The listing builds one solid part. Answer for the finished solid, in the listing's coordinates (mm). Give positions to 0.01 mm unless a question says otherwise; leave off trailing zeros. Order: outer loops, then holes, each group sorted by start corner. A loop starts at its lowest first (then second) coordinate and runs counter-clockwise, first axis right, second up. Notation, with made-up numbers: M 29.25,24.25 L 65.25,24.25 A15 ccw 65.25,46.25 Z; hole C 65.5,81.5 d1. An arc over 180 degrees is marked long. Answer as a JSON object with one key per item and string values. Group by question number.
```python
from build123d import *

# Parameters (mm, degrees)
SKETCH_1_R      = 0.4
EXTRUDE_1_DEPTH = 10
SKETCH_2_W      = 80
SKETCH_2_H      = 0.8
EXTRUDE_2_DEPTH = 0.8
FILLET_1_R      = 0.4
SKETCH_3_R      = 0.4
EXTRUDE_3_DEPTH = 4
SKETCH_4_R      = 0.4
EXTRUDE_4_DEPTH = 4


with BuildPart() as part:
    # 草图1 → 凸台-拉伸1 (new body)
    with BuildSketch(Plane(origin=(0, 0, 0), x_dir=(1, 0, 0), z_dir=(0, 1, 0))):
        with Locations(Location((0, 0, 0), (0, 0, 270))):
            Circle(SKETCH_1_R)
    extrude(amount=EXTRUDE_1_DEPTH)

    # 草图2 → 凸台-拉伸2 (add)
    with BuildSketch(Plane(origin=(0, 10, 0), x_dir=(1, 0, 0), z_dir=(0, 1, 0))):
        Rectangle(SKETCH_2_W, SKETCH_2_H)
    extrude(amount=EXTRUDE_2_DEPTH)

    # 圆角1
    fillet_1_edges = [part.edges().sort_by_distance(p)[0] for p in [
        (40, 10, 0),
        (40, 10.8, 0),
        (-40, 10, 0),
        (-40, 10.8, 0),
    ]]
    fillet(fillet_1_edges, radius=FILLET_1_R - 0.0001)  # a hair under: the kernel refuses the full size

    # 草图3 → 凸台-拉伸3 (add)
    with BuildSketch(Plane.XY.offset(0.4)):
        with Locations((39.6, 10.4)):
            Circle(SKETCH_3_R)
    extrude(amount=EXTRUDE_3_DEPTH)

    # 草图4 → 凸台-拉伸4 (add)
    with BuildSketch(Plane(origin=(0, 0, -0.4), x_dir=(-1, 0, 0), z_dir=(0, 0, -1))):
        with Locations((39.6, 10.4)):
            Circle(SKETCH_4_R)
    extrude(amount=EXTRUDE_4_DEPTH)

    # 草图5 → 旋转1 (revolve)
    with BuildSketch(Plane(origin=(0, 10.4, 0), x_dir=(1, 0, 0), z_dir=(0, 1, 0))):
        Polygon((39.6, -4.4), (39.6, -5.4), (40, -4.4), align=None)
    revolve(axis=Axis((39.6, 10.4, 4.4), (0, 0, 1)))

    # 草图6 → 旋转2 (revolve)
    with BuildSketch(Plane(origin=(0, 10.4, 0), x_dir=(1, 0, 0), z_dir=(0, 1, 0))):
        Polygon((-39.6, 4.4), (-39.6, 5.4), (-40, 4.4), align=None)
    revolve(axis=Axis((-39.6, 10.4, -4.4), (0, 0, -1)))


solid = part.part
```
Item 1: Section C-C (y = 2.5) is taken. Determine the outline of the cut face in (x, z), and give its area (3 significant figures).
Item 2: Consider probe 1 along Y at (x, z) = (4, 0). Determine where the line is inside the solid, lowest interval first. Write a range as from..to.
Item 3: Section A-A (z = 3.5) is taken. Determine the outline of the cut face in (x, y), and give its area (3 significant figures).
Item 4: Section B-B (x = 14.5) is taken. Determine the outline of the cut face in (y, z), and give its area (3 significant figures).
Item 5: A flat-ended cylindrical pin translates along its axis: P1, Ø0.6, axis at x = 15, z = 0, coming from the -Y side. Find the tip coordinate at first contact, or state that the pin passes through.
Values found:
{
 "1": {"outline": "C 0,0 d0.8", "area": "0.503 mm^2"},
 "2": {"probe 1": "y = 10..10.8"},
 "3": {"outline": "C 39.6,10.4 d0.8", "area": "0.503 mm^2"},
 "4": {"outline": "M 10,-0.4 L 10.8,-0.4 L 10.8,0.4 L 10,0.4 Z", "area": "0.640 mm^2"},
 "5": {"P1": "stops at y = 10"}
}
